Geometry: final body of the model. Coordinates: model frame, mm. Give positions to 0.01 mm unless a question says otherwise; leave off trailing zeros. Write each loop counter-clockwise with the first axis right and the second up, starting at its lowest first coordinate (ties: lowest second). Pieces come first, ordered by that corner, then holes.
```python
from build123d import *

# Parameters (mm, degrees)
F1_R     = 3.25
F1_R_2   = 2.75
F2_DEPTH = 3.125


with BuildPart() as f2:
    # F1 (on Right) → F2 (new body)
    with BuildSketch(Plane.YZ):
        with BuildLine():
            Line((10, 43.757633), (-10, 43.757633))
            ThreePointArc((-10, 43.757633), (-16.160663, 41.870603), (-20.207625, 36.856948))
            Line((-20.207625, 36.856948), (-33.063557, 4.844646))
            ThreePointArc((-33.063557, 4.844646), (-31.769875, -7.280783), (-21, -13))
            Line((-21, -13), (21, -13))
            ThreePointArc((21, -13), (31.769875, -7.280783), (33.063557, 4.844646))
            Line((33.063557, 4.844646), (20.207625, 36.856948))
            ThreePointArc((20.207625, 36.856948), (16.160663, 41.870603), (10, 43.757633))
        make_face()
        with Locations((-21, 0)):
            Circle(F1_R, mode=Mode.SUBTRACT)
        with Locations((21, 0)):
            Circle(F1_R, mode=Mode.SUBTRACT)
        with Locations((-10, 32.757633)):
            Circle(F1_R_2, mode=Mode.SUBTRACT)
        with Locations((10, 32.757633)):
            Circle(F1_R_2, mode=Mode.SUBTRACT)
    extrude(amount=F2_DEPTH)


solid = f2.part
```
Item 1: Line query: L1, parallel to Y at x = 2.75, z = 0.5; L2, parallel to Z at x = 2.05, y = 10; L3, parallel to Z at x = 2.75, y = -21. Output: solid intervals per line, ascending.
Found:
L1: y = -33.99 to -24.21, -17.79 to 17.79, 24.21 to 33.99
L2: z = -13 to 30.01, 35.51 to 43.76
L3: z = -13 to -3.25, 3.25 to 34.88
Item 2: Section A-A, the plane z = 0. Return the cut outline in (x, y) (3 decimals), plus the area to 3 significant figures.
Found:
outline: (0, -34) - (3.125, -34) - (3.125, -24.25) - (0, -24.25) - close; (0, -17.75) - (3.125, -17.75) - (3.125, 17.75) - (0, 17.75) - close; (0, 24.25) - (3.125, 24.25) - (3.125, 34) - (0, 34) - close
area: 172 mm2
Item 3: Pull-direction query (Z, two-part tool) for faces 1 (the face through (1.541, 17.753, 0.143)), 2 (the face through (3.125, 0, 16)), 3 (the face through (1.541, -24.247, 0.143)), 4 (the face through (1.541, -16.085, 41.922)); classes: +Z half, -Z half, draft (parallel to the pull), parting line (faces both ways), or undercut.
Found:
face 1: undercut
face 2: draft
face 3: undercut
face 4: +Z half
Item 4: Section C-C, the plane y = -29. Return the cut outline in (x, z) (3 decimals), plus the area to 3 significant figures.
Found:
outline: (0, -10.247) - (3.125, -10.247) - (3.125, 14.963) - (0, 14.963) - close
area: 78.8 mm2
Item 5: Section B-B, the plane x = 0.5. Return the cut outline in (y, z), plus the area to 3 significant figures.
Found:
outline: (-33.06, 4.84) arc R13 ccw to (-21, -13) - (21, -13) arc R13 ccw to (33.06, 4.84) - (20.21, 36.86) arc R11 ccw to (10, 43.76) - (-10, 43.76) arc R11 ccw to (-20.21, 36.86) - close; hole circle Ø6.5 at (-21, 0); hole circle Ø5.5 at (-10, 32.76); hole circle Ø5.5 at (10, 32.76); hole circle Ø6.5 at (21, 0)
area: 2,970 mm2
Item 6: Section D-D, the plane z = 27. Return the cut outline in (x, y) (3 decimals), plus the area to 3 significant figures.
Found:
outline: (0, -24.166) - (3.125, -24.166) - (3.125, 24.166) - (0, 24.166) - close
area: 151 mm2
